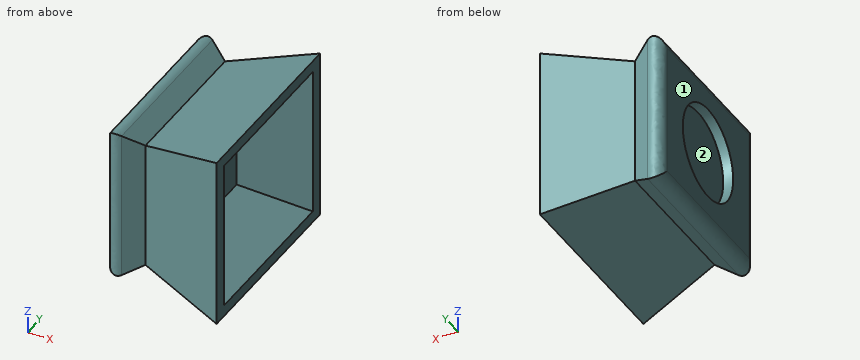
```python
from build123d import *

# Parameters (mm, degrees)
F0_W          = 44.3588159978
F0_H          = 38.4979620576
F1_DEPTH      = 25
F1_TAPER      = -15
F1_DEPTH_BACK = 10
F1_TAPER_BACK = -30
F2_W          = 49.5432667505
F2_H          = 45
F3_DEPTH      = 20
F3_TAPER      = 15
F4_R          = 3
F5_R          = 14.044270733
F6_DEPTH      = 3


with BuildPart() as f1:
    # F0 (on Right) → F1 (new body, two sides)
    with BuildSketch(Plane.YZ) as f1_sk:
        Rectangle(F0_W, F0_H)
    extrude(amount=F1_DEPTH, taper=F1_TAPER)
    extrude(f1_sk.sketch, amount=-F1_DEPTH_BACK, taper=F1_TAPER_BACK)

    # F2 (on face) → F3 (cut)
    with BuildSketch(Plane.YZ.offset(25)):
        Rectangle(F2_W, F2_H)
    extrude(amount=-F3_DEPTH, taper=F3_TAPER, mode=Mode.SUBTRACT)

    # F4
    f4_edges = [f1.edges().sort_by_distance(p)[0] for p in [
        (-10, 27.952911, 0),
        (-10, 0, 25.022484),
        (-10, -27.952911, 0),
        (-10, 0, -25.022484),
    ]]
    fillet(f4_edges, radius=F4_R)

    # F5 (on face) → F6 (cut)
    with BuildSketch(Plane(origin=(-10, 0, 0), x_dir=(0, -1, 0), z_dir=(-1, 0, 0))):
        Circle(F5_R)
    extrude(amount=-F6_DEPTH, mode=Mode.SUBTRACT)


solid = f1.part
```
CAD build for the part. Positions are in the model's coordinates, mm. Face numbers are marked on the shaded views. Coordinates: 2 decimals unless noted, no trailing zeros.
(1) Drill centre lines: L1, parallel to Z at x = -8.5, y = 0; L2, parallel to X at y = -7.5, z = 11; L3, parallel to Z at x = -8.65, y = 0. Where is each one in solid material? Low to high.
Solution:
L1: z = -22.42 to -14.04, 14.04 to 22.42
L2: x = -7 to 5
L3: z = -22.33 to -14.04, 14.04 to 22.33
(2) Pin check, flat tips, straight feed: pin 1 Ø1.5 at (y, z) = (2.5, 2.5) entering from -X; pin 2 Ø10.5 at (y, z) = (2, -7.5) entering from +X; pin 3 Ø1.5 at (x, z) = (18, -10.5) entering from +Y. Stop position of each tip, or through.
Solution:
pin 1: stops at x = -7
pin 2: stops at x = 5
pin 3: stops at y = 27.2
(3) Mould opens along Z. For the marked faces 1 and 2 say: released by +Z, released by -Z, zero draft, split by the parting line, or undercut.
Solution:
face 1: zero draft
face 2: undercut
